Drawing for the job (mm, zero at the part's lowest x, y, z). A direction names the side the tool comes from. Give positions to 0.01 mm unless a question says otherwise; leave off trailing zeros. Order: outer loops, then holes, each group sorted by start corner. A loop starts at its lowest first (then second) coordinate and runs counter-clockwise, first axis right, second up. Notation, with made-up numbers: M 60.25,18 L 101.25,18 A16 cw 101.25,29 Z; hole C -34.5,43.5 d4. An arc over 180 degrees is marked long. One line per item, written item: value.
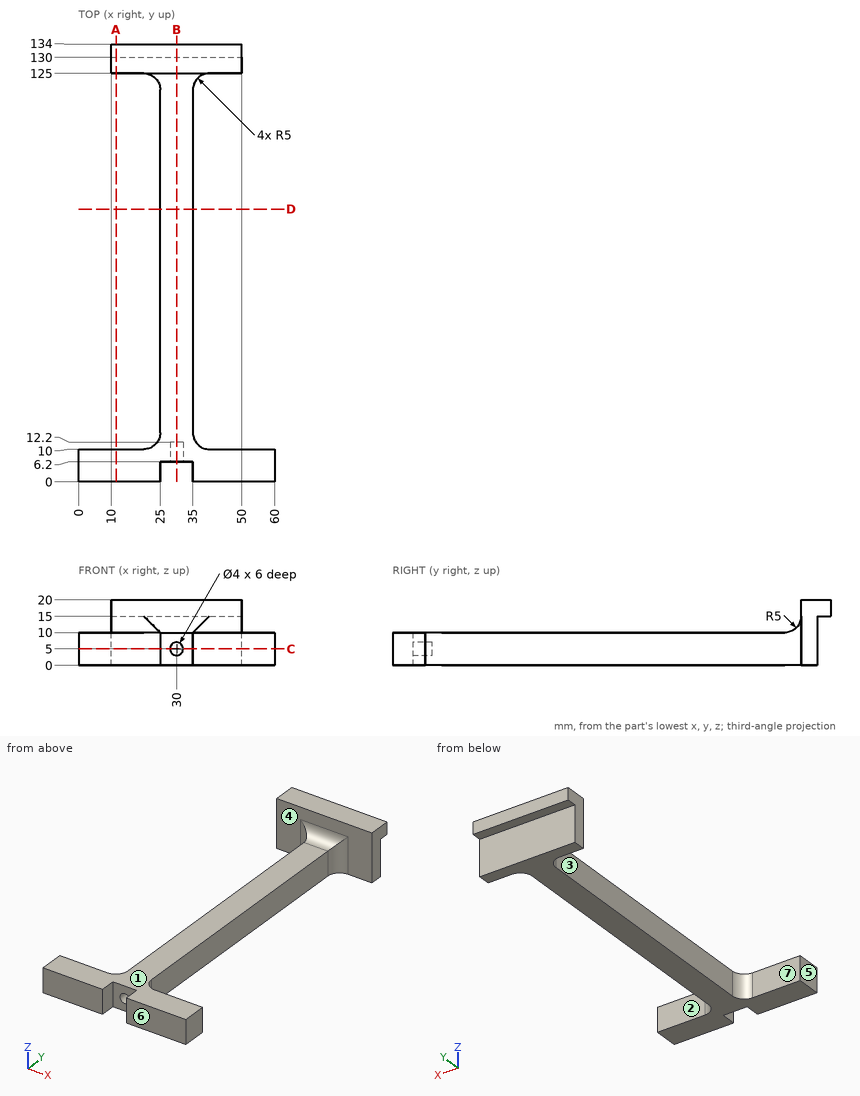
1) Pin check, flat tips, straight feed: pin 1 (4.5 mm diameter, centred on x = 30, z = 5, fed in from +Y); pin 2 (8 mm diameter, centred on x = 30.5, z = 4, fed in from -Y); pin 3 (6 mm diameter, centred on y = 66.5, z = 4.5, fed in from -X). Stop position of each tip, or through.
Check values:
pin 1: y = 130
pin 2: y = 6.2
pin 3: x = 25
2) Saw through at C-C, the plane z = 5. Write the cut outline in (x, y), then the cut area to 3 significant figures.
Check values:
outline: M 0,0 L 25,0 L 25,6.2 L 28,6.2 L 28,12.2 L 32,12.2 L 32,6.2 L 35,6.2 L 35,0 L 60,0 L 60,10 L 40,10 A5 cw 35,15 L 35,120 A5 cw 40,125 L 50,125 L 50,130 L 10,130 L 10,125 L 20,125 A5 cw 25,120 L 25,15 A5 cw 20,10 L 0,10 Z
area: 1,890 mm^2
3) Saw through at D-D, the plane y = 83.5. Write the cut outline in (x, z), then the cut area to 3 significant figures.
Check values:
outline: M 25,0 L 35,0 L 35,10 L 25,10 Z
area: 100 mm^2
4) Tool access for the marked faces 1, 2, 3 and 4: list every direction of +Z, -Z, +X, -X, +Y, -Y with a clear straight run to the whole face (end or side of a thin tool).
Check values:
face 1: +Z, +X, -X, -Y
face 2: +Z, -Z, +X
face 3: +Z, -Z, -X
face 4: +Z
5) Saw through at B-B, the plane x = 30. Write the cut outline in (y, z).
Check values:
outline: M 6.2,0 L 130,0 L 130,15 L 134,15 L 134,20 L 125,20 L 125,15 A5 cw 120,10 L 6.2,10 L 6.2,7 L 12.2,7 L 12.2,3 L 6.2,3 Z
6) Drill centre lines: probe 1 along Y at (x, z) = (46.5, 1.5); probe 2 along X at (y, z) = (9.25, 5); probe 3 along Y at (x, z) = (38.5, 18.5). Where is each one in solid material? Low to high. Write a range as from..to.
Check values:
probe 1: 0..10, 125..130
probe 2: 0..28, 32..60
probe 3: 125..134
7) Mould opens along Y. For the marked faces 5, 6 and 7 say: released by +Y, released by -Y, zero draft, split by the parting line, or undercut.
Check values:
face 5: zero draft
face 6: released by -Y
face 7: undercut
8) Saw through at A-A, the plane x = 11.5. Write the cut outline in (y, z).
Check values:
outline: M 0,0 L 10,0 L 10,10 L 0,10 Z; M 125,0 L 130,0 L 130,15 L 134,15 L 134,20 L 125,20 Z
